Build history of the part. All positions in model axes, mm. Face numbers are marked on the shaded views. A direction names the side the tool comes from. Coordinates: 2 decimals unless noted, no trailing zeros. Loops run counter-clockwise (first coordinate to the right, second up) from the corner with the lowest first, then second, coordinate; pieces in that order, holes last.
Item 1: 3-axis set-ups, long thin cutter, end or side, ignore diameter. For the marked faces 1 and 2: which of +Z, -Z, +X, -X, +Y, -Y reach the whole face in a straight line?
Item 2: Cut at C-C (z = 3.5). List the corners of the cut face in (x, y).
Item 3: Mould opens along Y. For the marked faces 3, 4 and 5 say: released by +Y, released by -Y, zero draft, split by the parting line, or undercut.
Item 4: Cut at D-D (x = -3). List the corners of the cut face in (y, z).
Item 5: Cut at A-A (y = 0). List the corners of the cut face in (x, z).
Item 6: Flat gauge pins, fed straight in: pin 1 (12 mm diameter, centred on x = 0.5, y = 0.5, fed in from +Z); pin 2 (3 mm diameter, centred on x = 19.5, z = 3.5, fed in from -Y); pin 3 (1.2 mm diameter, centred on x = 14, z = 4.5, fed in from +Y); pin 4 (6 mm diameter, centred on x = 0, y = -15, fed in from +Z). Where does each tip first touch, or does it go through?
Item 7: Cut at B-B (x = 25). List the corners of the cut face in (y, z).
Item 8: Drill centre lines: line 1 along Y through (x, z) = (0, 4.1); line 2 along Y through (x, z) = (-5, 4.7); line 3 along Y through (x, z) = (0, 1.15). Where is each one in solid material? Low to high.
from build123d import *

# Parameters (mm, degrees)
SKETCH1_R           = 2.5
BOSS_EXTRUDE1_DEPTH = 6
CUT_EXTRUDE1_REACH  = 51.608
SKETCH2_W           = 4
SKETCH2_H           = 20
CUT_EXTRUDE2_REACH  = 42.509
SKETCH3_R           = 3.1


with BuildPart() as part:
    # Sketch1 → Boss-Extrude1 (new body)
    with BuildSketch(Plane.XY):
        Polygon((10, 20), (35, 12.5), (35, -12.5), (10, -20), (-10, -20), (-10, 20), align=None)
        with Locations((0, -15)):
            Circle(SKETCH1_R, mode=Mode.SUBTRACT)
        with Locations((0, 15)):
            Circle(SKETCH1_R, mode=Mode.SUBTRACT)
    extrude(amount=BOSS_EXTRUDE1_DEPTH)

    # Sketch2 → Cut-Extrude1 (cut, up to next)
    with BuildSketch(Plane(origin=(35, 0, 0), x_dir=(0, 0, -1), z_dir=(1, 0, 0)), mode=Mode.PRIVATE) as cut_extrude1_sk1:
        with Locations((-4, 0)):
            Rectangle(SKETCH2_W, SKETCH2_H)
    cut_extrude1_tool1 = extrude(cut_extrude1_sk1.sketch, amount=-CUT_EXTRUDE1_REACH, mode=Mode.PRIVATE) & part.part
    add(cut_extrude1_tool1.solids().sort_by_distance((35, 0, 4))[0], mode=Mode.SUBTRACT)

    # Sketch3 → Cut-Extrude2 (cut, up to next)
    with BuildSketch(Plane.XY.offset(2), mode=Mode.PRIVATE) as cut_extrude2_sk1:
        with Locations((25, 0)):
            Circle(SKETCH3_R)
    cut_extrude2_tool1 = extrude(cut_extrude2_sk1.sketch, amount=-CUT_EXTRUDE2_REACH, mode=Mode.PRIVATE) & part.part
    add(cut_extrude2_tool1.solids().sort_by_distance((25, 0, 2))[0], mode=Mode.SUBTRACT)


solid = part.part
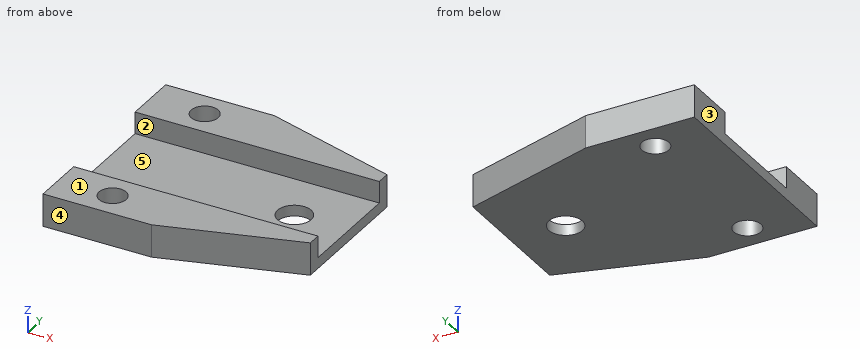
Filled sheet:
1. face 1: +Z, +X, -X, +Y, -Y
1. face 2: +Z, +X, -X
2. outline: (-10, -20) - (10, -20) - (35, -12.5) - (35, -10) - (-10, -10) - close; (-10, 10) - (35, 10) - (35, 12.5) - (10, 20) - (-10, 20) - close; hole circle Ø5 at (0, -15); hole circle Ø5 at (0, 15)
3. face 3: zero draft
3. face 4: released by -Y
3. face 5: undercut
4. outline: (-20, 0) - (20, 0) - (20, 6) - (10, 6) - (10, 2) - (-10, 2) - (-10, 6) - (-20, 6) - close
5. outline: (-10, 0) - (21.9, 0) - (21.9, 2) - (-10, 2) - close; (28.1, 0) - (35, 0) - (35, 2) - (28.1, 2) - close
6. pin 1: stops at z = 2
6. pin 2: stops at y = -17.6
6. pin 3: stops at y = 18.98
6. pin 4: stops at z = 6
7. outline: (-15.5, 0) - (-3.1, 0) - (-3.1, 2) - (-10, 2) - (-10, 6) - (-15.5, 6) - close; (3.1, 0) - (15.5, 0) - (15.5, 6) - (10, 6) - (10, 2) - (3.1, 2) - close
8. line 1: y = -20 to -17.5, -12.5 to -10, 10 to 12.5, 17.5 to 20
8. line 2: y = -20 to -10, 10 to 20
8. line 3: y = -20 to -17.5, -12.5 to 12.5, 17.5 to 20
